Geometry check sheet. Reference: the model listing, model coordinates, mm. Face numbers are marked on the shaded views. Coordinates: 2 decimals unless noted, no trailing zeros. Write each loop counter-clockwise with the first axis right and the second up, starting at its lowest first coordinate (ties: lowest second). Pieces come first, ordered by that corner, then holes.
from build123d import *

# Parameters (mm, degrees)
SKETCH1_R           = 6
BOSS_EXTRUDE1_DEPTH = 5
SKETCH2_R           = 2.5
BOSS_EXTRUDE2_DEPTH = 12
SKETCH4_W           = 0.625
SKETCH4_H           = 0.5


with BuildPart() as part:
    # Sketch1 → Boss-Extrude1 (new body)
    with BuildSketch(Plane(origin=(0, 0, 0), x_dir=(1, 0, 0), z_dir=(0, 1, 0))):
        with Locations(Location((0, 0, 0), (0, 0, 270))):
            Circle(SKETCH1_R)
    extrude(amount=BOSS_EXTRUDE1_DEPTH)

    # Sketch2 → Boss-Extrude2 (add)
    with BuildSketch(Plane(origin=(0, 5, 0), x_dir=(-1, 0, 0), z_dir=(0, 1, 0))):
        with Locations(Location((0, 0, 0), (0, 0, 90))):
            Circle(SKETCH2_R)
    extrude(amount=-BOSS_EXTRUDE2_DEPTH)

    # Sketch4 → Groove for ANSI B27.7 - 3AM1-5, Basic External Retaining Ring1 (revolve, cut)
    with BuildSketch(Plane(origin=(0, -7, 0), x_dir=(0, 0, 1), z_dir=(-1, 0, 0))):
        with Locations((2.6875, 0.751696416)):
            Rectangle(SKETCH4_W, SKETCH4_H)
    revolve(axis=Axis((0, -57, 0), (0, 1, 0)), mode=Mode.SUBTRACT)


solid = part.part
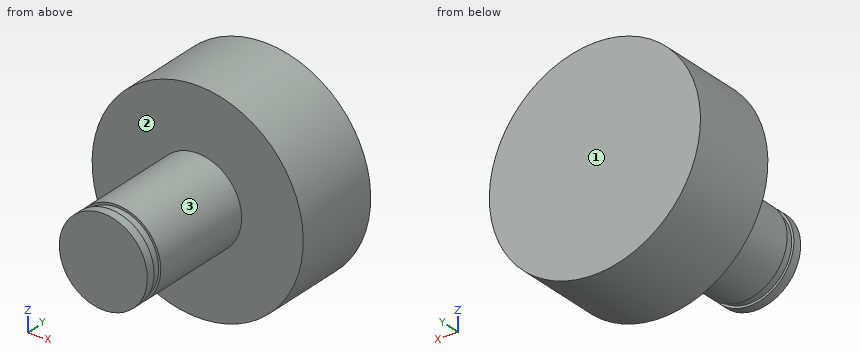
1. Sectioned sample at A-A, the plane x = 0. Record the boundary of the cut face in (y, z) (3 decimals), and give its area (3 significant figures).
Computed values:
outline: (-7, -2.5) - (-6.498, -2.5) - (-6.498, -2.375) - (-5.998, -2.375) - (-5.998, -2.5) - (0, -2.5) - (0, -6) - (5, -6) - (5, 6) - (0, 6) - (0, 2.5) - (-5.998, 2.5) - (-5.998, 2.375) - (-6.498, 2.375) - (-6.498, 2.5) - (-7, 2.5) - close
area: 94.9 mm2
2. Draft check along Y on the marked faces 1, 2 and 3. Enter one of: released by +Y, released by -Y, zero draft, split by the parting line, or undercut.
Computed values:
face 1: released by +Y
face 2: released by -Y
face 3: zero draft
3. Sectioned sample at C-C, the plane y = -0.75. Record the boundary of the cut face in (x, z), and give its area (3 significant figures).
Computed values:
outline: circle Ø5 at (0, 0)
area: 19.6 mm2
4. Thickness scan on line 1 along Y through (x, z) = (0.5, 3.75); line 2 along X through (y, z) = (-4.5, 0); line 3 along X through (y, z) = (1.25, -2.5). Record the ranges inside material, lowest first.
Computed values:
line 1: y = 0 to 5
line 2: x = -2.5 to 2.5
line 3: x = -5.45 to 5.45
5. Gauge pin test, flat ends, axial feed: pin 1 Ø3 at (x, y) = (0, -2.5) entering from -Z; pin 2 Ø6 at (x, y) = (3.5, -0.5) entering from +Z; pin 3 Ø1 at (x, z) = (3, -0.5) entering from -Y. Record the tip position at first contact, or that the pin passes through.
Computed values:
pin 1: stops at z = -2.5
pin 2: stops at z = 5.98
pin 3: stops at y = 0
6. Sectioned sample at D-D, the plane z = -3.5. Record the boundary of the cut face in (x, y).
Computed values:
outline: (-4.87, 0) - (4.87, 0) - (4.87, 5) - (-4.87, 5) - close
7. Sectioned sample at B-B, the plane z = 0. Record the boundary of the cut face in (x, y) (3 decimals).
Computed values:
outline: (-6, 0) - (-2.5, 0) - (-2.5, -5.998) - (-2.375, -5.998) - (-2.375, -6.498) - (-2.5, -6.498) - (-2.5, -7) - (2.5, -7) - (2.5, -6.498) - (2.375, -6.498) - (2.375, -5.998) - (2.5, -5.998) - (2.5, 0) - (6, 0) - (6, 5) - (-6, 5) - close
